Build history of the part. All positions in model axes, mm. Round coordinates to 2 decimals unless told otherwise and drop trailing zeros. Order: outer loops, then holes, each group sorted by start corner. A loop starts at its lowest first (then second) coordinate and runs counter-clockwise, first axis right, second up. Notation, with made-up numbers: (-3.5, 26) -> (36.5, 26) arc R32 cw to (36.5, 65) -> close; hole circle Ø3 at (66, -39). An arc over 180 degrees is marked (long way). Use a Markdown table: item, result. Add a question column.
Item 1: Slice it at B-B, the plane z = 16. Give the cut face in (x, y).
Item 2: Slice it at D-D, the plane x = 0.5. Give the cut face in (y, z), plus the area to 3 significant figures.
Item 3: Probe L1, parallel to Z at x = 1.3, y = -17.5; L2, parallel to Y at x = 0.4, z = -5; L3, parallel to Z at x = 1.4, y = 38.5. List the from-to ranges inside material, lowest first.
Item 4: Slice it at A-A, the plane z = -1.5. Give the cut face in (x, y), plus the area to 3 significant figures.
Item 5: Slice it at C-C, the plane y = 17.5. Give the cut face in (x, z), plus the area to 3 significant figures.
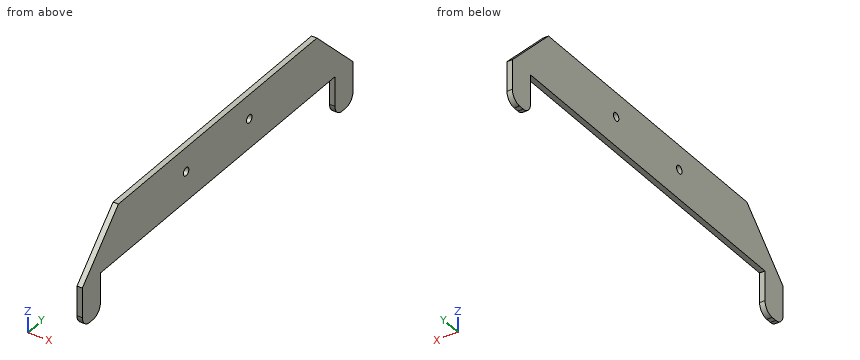
from build123d import *

# Parameters (mm, degrees)
SKETCH018_W     = 150
SKETCH018_H     = 35
PAD010_DEPTH    = 2
SKETCH019_W     = 130
SKETCH019_H     = 50
POCKET007_DEPTH = 2
FILLET_R        = 4
SKETCH020_R     = 1.5
POCKET008_DEPTH = 2
CHAMFER002_SIZE = 20


with BuildPart() as part:
    # Sketch018 → Pad010 (new body)
    with BuildSketch(Plane.YZ):
        with Locations((0, 7.5)):
            Rectangle(SKETCH018_W, SKETCH018_H)
    extrude(amount=PAD010_DEPTH)

    # Sketch019 → Pocket007 (cut)
    with BuildSketch(Plane.YZ):
        with Locations((0, -20)):
            Rectangle(SKETCH019_W, SKETCH019_H)
    extrude(amount=POCKET007_DEPTH, mode=Mode.SUBTRACT)

    # Fillet
    fillet_edges = [part.edges().sort_by_distance(p)[0] for p in [
        (1, -65, -10),
        (1, -75, -10),
        (1, 65, -10),
        (1, 75, -10),
    ]]
    fillet(fillet_edges, radius=FILLET_R)

    # Sketch020 → Pocket008 (cut)
    with BuildSketch(Plane.YZ):
        with Locations((17.5, 16)):
            Circle(SKETCH020_R)
        with Locations((-17.5, 16)):
            Circle(SKETCH020_R)
    extrude(amount=POCKET008_DEPTH, mode=Mode.SUBTRACT)

    # Chamfer002
    chamfer002_edges = [part.edges().sort_by_distance(p)[0] for p in [
        (1, -75, 25),
        (1, 75, 25),
    ]]
    chamfer(chamfer002_edges, length=CHAMFER002_SIZE)


solid = part.part
Check sheet entries:
| question | item | result |
|---|---|---|
| 1 | outline | (0, -64) -> (2, -64) -> (2, -19) -> (0, -19) -> close; (0, -16) -> (2, -16) -> (2, 16) -> (0, 16) -> close; (0, 19) -> (2, 19) -> (2, 64) -> (0, 64) -> close |
| 2 | outline | (-75, -6) arc R4 ccw to (-71, -10) -> (-69, -10) arc R4 ccw to (-65, -6) -> (-65, 5) -> (65, 5) -> (65, -6) arc R4 ccw to (69, -10) -> (71, -10) arc R4 ccw to (75, -6) -> (75, 5) -> (55, 25) -> (-55, 25) -> (-75, 5) -> close; hole circle Ø3 at (-17.5, 16); hole circle Ø3 at (17.5, 16) |
| 2 | area | 2,870 mm2 |
| 3 | L1 | 5 to 14.5, 17.5 to 25 |
| 3 | L2 | -75 to -65, 65 to 75 |
| 3 | L3 | 5 to 25 |
| 4 | outline | (0, -75) -> (2, -75) -> (2, -65) -> (0, -65) -> close; (0, 65) -> (2, 65) -> (2, 75) -> (0, 75) -> close |
| 4 | area | 40.0 mm2 |
| 5 | outline | (0, 5) -> (2, 5) -> (2, 14.5) -> (0, 14.5) -> close; (0, 17.5) -> (2, 17.5) -> (2, 25) -> (0, 25) -> close |
| 5 | area | 34.0 mm2 |
